```python
from build123d import *

# Parameters (mm, degrees)
SKETCH1_W           = 80
SKETCH1_H           = 80
BOSS_EXTRUDE1_DEPTH = 25.3
SKETCH2_R           = 38
CUT_EXTRUDE1_DEPTH  = 25.3
SKETCH4_R           = 2
CUT_EXTRUDE2_DEPTH  = 25.3
SKETCH9_R           = 2
CUT_EXTRUDE3_DEPTH  = 25.3
SKETCH10_W          = 4.103880803
SKETCH10_H          = 80
SKETCH10_W_2        = 4
BOSS_EXTRUDE2_DEPTH = 1.37
SKETCH11_W          = 2.051940402
SKETCH11_H          = 80
BOSS_EXTRUDE3_DEPTH = 10
SKETCH12_W          = 2
SKETCH12_H          = 80
BOSS_EXTRUDE4_DEPTH = 10


with BuildPart() as part:
    # Sketch1 → Boss-Extrude1 (new body)
    with BuildSketch(Plane(origin=(0, 0, 0), x_dir=(0, 0, -1), z_dir=(1, 0, 0))):
        with Locations((2.081688293, -16.943070175)):
            Rectangle(SKETCH1_W, SKETCH1_H)
    extrude(amount=BOSS_EXTRUDE1_DEPTH)

    # Sketch2 → Cut-Extrude1 (cut)
    with BuildSketch(Plane(origin=(25.3, 0, 0), x_dir=(0, 0, -1), z_dir=(1, 0, 0))):
        with Locations((2.081688293, -16.943070175)):
            Circle(SKETCH2_R)
    extrude(amount=-CUT_EXTRUDE1_DEPTH, mode=Mode.SUBTRACT)

    # Sketch4 → Cut-Extrude2 (cut)
    with BuildSketch(Plane.ZY):
        with Locations((-38.081688293, 19.056929825)):
            Circle(SKETCH4_R)
    extrude(amount=-CUT_EXTRUDE2_DEPTH, mode=Mode.SUBTRACT)

    # Sketch9 → Cut-Extrude3 (cut)
    with BuildSketch(Plane.ZY):
        with Locations((33.918311707, 19.056929825)):
            Circle(SKETCH9_R)
        with Locations((33.918311707, -52.943070175)):
            Circle(SKETCH9_R)
        with Locations((-38.081688293, -53.283129164)):
            Circle(SKETCH9_R)
    extrude(amount=-CUT_EXTRUDE3_DEPTH, mode=Mode.SUBTRACT)

    # Sketch10 → Boss-Extrude2 (add)
    with BuildSketch(Plane(origin=(25.3, 0, 0), x_dir=(0, 0, -1), z_dir=(1, 0, 0))):
        with Locations((-35.866371306, -16.943070175)):
            Rectangle(SKETCH10_W, SKETCH10_H)
        with Locations((40.081688293, -16.943070175)):
            Rectangle(SKETCH10_W_2, SKETCH10_H)
    extrude(amount=BOSS_EXTRUDE2_DEPTH)

    # Sketch11 → Boss-Extrude3 (add)
    with BuildSketch(Plane(origin=(26.67, 0, 0), x_dir=(0, 0, -1), z_dir=(1, 0, 0))):
        with Locations((-36.892341506, -16.943070175)):
            Rectangle(SKETCH11_W, SKETCH11_H)
    extrude(amount=BOSS_EXTRUDE3_DEPTH)

    # Sketch12 → Boss-Extrude4 (add)
    with BuildSketch(Plane(origin=(26.67, 0, 0), x_dir=(0, 0, -1), z_dir=(1, 0, 0))):
        with Locations((41.081688293, -16.943070175)):
            Rectangle(SKETCH12_W, SKETCH12_H)
    extrude(amount=BOSS_EXTRUDE4_DEPTH)


solid = part.part
```
CAD build for the part. Positions are in the model's coordinates, mm. A direction names the side the tool comes from. Round coordinates to 2 decimals unless told otherwise and drop trailing zeros. Order: outer loops, then holes, each group sorted by start corner. A loop starts at its lowest first (then second) coordinate and runs counter-clockwise, first axis right, second up.
Q1. Which spindle directions (+Z, -Z, +X, -X, +Y, -Y) get a long thin tool onto all of the face, cutting with end or side? Do faces 1 (the cylindrical face through (12.47, -54.5, -39.67)), 2 (the flat face through (32, -18, 35.866)), 3 (the flat face through (36.67, -16, -41)). Say none if no direction does.
Q2. Wall check: L1, parallel to Z at x = 27.5, y = -1.5; L2, parallel to Y at x = 17, z = -27.5; L3, parallel to Y at x = 15.5, z = 5.5. Give the ranges that are in metal, low to high.
Q3. Slice it at D-D (y = 15). Write the cut outline in (x, z), and give its area (3 significant figures).
Q4. Drop flat-ended pins along their axis: pin 1 (3 mm diameter, centred on y = -52.94, z = 33.92, fed in from +X); pin 2 (1.7 mm diameter, centred on y = 18.5, z = 34.5, fed in from -X). Give the stop position or say it passes through.
Q5. Two-plate mould, pull along Y, no slides. Class faces 4 (the flat face through (26.67, -16, -39)), 5 (the flat face through (25.3, -17, 35)), 6 (the flat face through (14, 23.057, -2)), 7 (the flat face through (14, -56.943, -2)): pulls with the +Y half, pulls with the -Y half, needs draft (parallel to the pull), parting line crosses it, or undercut.
Q6. Slice it at A-A (x = 30). Write the cut outline in (y, z), and give its area (3 significant figures).
Q7. Slice it at B-B (z = 13.5). Write the cut outline in (x, y).
Q8. Slice it at C-C (y = -34). Write the cut outline in (x, z), and give its area (3 significant figures).
Results below:
1. face 1: -X
1. face 2: +X, +Y, -Y
1. face 3: +Z, -Z, +X, +Y, -Y
2. L1: z = -42.08 to -40.08, 35.87 to 37.92
2. L2: y = -56.94 to -45.19, 11.3 to 23.06
2. L3: y = -56.94 to -54.18, 20.29 to 23.06
3. outline: (0, -42.08) - (36.67, -42.08) - (36.67, -40.08) - (26.67, -40.08) - (26.67, -38.08) - (25.3, -38.08) - (25.3, -22.66) - (0, -22.66) - close; (0, 18.5) - (25.3, 18.5) - (25.3, 33.81) - (26.67, 33.81) - (26.67, 35.87) - (36.67, 35.87) - (36.67, 37.92) - (0, 37.92) - close
3. area: 1,030 mm2
4. pin 1: stops at x = 26.67
4. pin 2: stops at x = 25.3
5. face 4: needs draft
5. face 5: undercut
5. face 6: pulls with the +Y half
5. face 7: pulls with the -Y half
6. outline: (-56.94, -42.08) - (23.06, -42.08) - (23.06, -40.08) - (-56.94, -40.08) - close; (-56.94, 35.87) - (23.06, 35.87) - (23.06, 37.92) - (-56.94, 37.92) - close
6. area: 324 mm2
7. outline: (0, -56.94) - (25.3, -56.94) - (25.3, -51.6) - (0, -51.6) - close; (0, 17.72) - (25.3, 17.72) - (25.3, 23.06) - (0, 23.06) - close
8. outline: (0, -42.08) - (36.67, -42.08) - (36.67, -40.08) - (26.67, -40.08) - (26.67, -38.08) - (25.3, -38.08) - (25.3, -36.04) - (0, -36.04) - close; (0, 31.88) - (25.3, 31.88) - (25.3, 33.81) - (26.67, 33.81) - (26.67, 35.87) - (36.67, 35.87) - (36.67, 37.92) - (0, 37.92) - close
8. area: 357 mm2
